```python
from build123d import *

# Parameters (mm, degrees)
EXTRUSION1_DEPTH = 267
ESQUISSE2_R      = 1.5
EXTRUSION2_DEPTH = 269.38638192
ESQUISSE3_R      = 1.5
EXTRUSION3_DEPTH = 264


with BuildPart() as part:
    # Esquisse1 → Extrusion1 (new body)
    with BuildSketch(Plane.XY):
        Polygon((0, 0), (20, 0), (20, 1.5), (1.5, 1.5), (1.5, 20), (0, 20), align=None)
    extrude(amount=EXTRUSION1_DEPTH)

    # Esquisse2 → Extrusion2 (cut, through all)
    with BuildSketch(Plane(origin=(0, 1.5, 0), x_dir=(1, 0, 0), z_dir=(0, 1, 0))):
        with Locations(Location((10, -30, 0), (0, 0, 180))):
            Circle(ESQUISSE2_R)
        with Locations(Location((10, -237, 0), (0, 0, 180))):
            Circle(ESQUISSE2_R)
    extrude(amount=-EXTRUSION2_DEPTH, mode=Mode.SUBTRACT)

    # Esquisse3 → Extrusion3 (cut)
    with BuildSketch(Plane(origin=(1.5, 0, 0), x_dir=(0, 0, -1), z_dir=(1, 0, 0))):
        with Locations(Location((-257, 10, 0), (0, 0, 90))):
            Circle(ESQUISSE3_R)
        with Locations(Location((-10, 10, 0), (0, 0, 90))):
            Circle(ESQUISSE3_R)
    extrude(amount=-EXTRUSION3_DEPTH, mode=Mode.SUBTRACT)


solid = part.part
```
For this review, take the finished solid that the model builds, in its own axes (mm). A direction names the side the tool comes from. Round coordinates to 2 decimals unless told otherwise and drop trailing zeros. Loops run counter-clockwise (first coordinate to the right, second up) from the corner with the lowest first, then second, coordinate; pieces in that order, holes last.
(1) We need section B-B (y = 4.25). Give the boundary of the cut face in (x, z).
Returned:
outline: (0, 0) - (1.5, 0) - (1.5, 267) - (0, 267) - close
(2) Wall thickness on line 1 along Z through (x, y) = (10, 1.1); line 2 along Z through (x, y) = (1, 10); line 3 along Y through (x, z) = (0.55, 257): over which ranges is each line inside the solid? List them lowest first.
Returned:
line 1: z = 0 to 28.5, 31.5 to 235.5, 238.5 to 267
line 2: z = 0 to 8.5, 11.5 to 255.5, 258.5 to 267
line 3: y = 0 to 8.5, 11.5 to 20
(3) Tool access review of faces 1 (the flat face through (0, 10, 132)), 2 (the flat face through (1.5, 11, 132)): name each direction out of +Z, -Z, +X, -X, +Y, -Y from which nothing blocks a thin tool from reaching the whole face with its end or side.
Returned:
face 1: +Z, -Z, -X, +Y, -Y
face 2: +Z, -Z, +X, +Y
(4) Clearance check with flat-ended pins moving along their axes: P1, Ø6, axis at y = 17, z = 101, coming from the +X side; P2, Ø1.5, axis at x = 17, z = 155, coming from the +Y side. State where each tip first meets the part, or that it passes through.
Returned:
P1: stops at x = 1.5
P2: stops at y = 1.5
(5) We need section A-A (z = 147). Give the boundary of the cut face in (x, y).
Returned:
outline: (0, 0) - (20, 0) - (20, 1.5) - (1.5, 1.5) - (1.5, 20) - (0, 20) - close
